```python
from build123d import *

# Parameters (mm, degrees)
BOSS_EXTRUDE1_DEPTH         = 35
CUT_EXTRUDE1_REACH          = 51.749
SKETCH2_R                   = 18
CUT_EXTRUDE2_DEPTH          = 22
CUT_EXTRUDE3_DEPTH          = 16
SKETCH5_W                   = 4.5
SKETCH5_H                   = 3
CUT_REVOLVE1_ANGLE          = 120
FILLET2_R                   = 1.5
CUT_EXTRUDE7_DEPTH          = 6.5
M3X0_25_TAPPED_HOLE1_REACH  = 71.769
M3X0_25_TAPPED_HOLE1_BORE_R = 1.375
M3X0_25_TAPPED_HOLE2_REACH  = 71.769
M3X0_25_TAPPED_HOLE2_BORE_R = 1.375
CUT_EXTRUDE8_REACH          = 71.769
CUT_EXTRUDE8_END_RADIUS     = 18
SKETCH15_R                  = 1.6
CUT_EXTRUDE9_REACH          = 71.769
CUT_EXTRUDE9_END_RADIUS     = 18
SKETCH16_R                  = 1.6
M5_TAPPED_HOLE3_D           = 4.2
M5_TAPPED_HOLE3_DEPTH       = 4.3
M5_TAPPED_HOLE3_TIP         = 1.2618073
M5_TAPPED_HOLE4_D           = 4.2
M5_TAPPED_HOLE4_DEPTH       = 4.3
M5_TAPPED_HOLE4_TIP         = 1.2618073
M3_TAPPED_HOLE1_D           = 2.5
M3_TAPPED_HOLE1_DEPTH       = 11.5
M3_TAPPED_HOLE1_TIP         = 0.751075774
FILLET3_R                   = 1.5


with BuildPart() as part:
    # Sketch1 → Boss-Extrude1 (new body)
    with BuildSketch(Plane(origin=(0, 0, 0), x_dir=(1, 0, 0), z_dir=(0, 1, 0))):
        Polygon((10.355339059, 25), (-10.355339059, 25), (-25, 10.355339059), (-25, -10.355339059), (-10.355339059, -25), (10.355339059, -25), (25, -10.355339059), (25, 10.355339059), align=None)
    extrude(amount=BOSS_EXTRUDE1_DEPTH)

    # Sketch2 → Cut-Extrude1 (cut, up to next)
    with BuildSketch(Plane(origin=(0, 35, 0), x_dir=(1, 0, 0), z_dir=(0, 1, 0)), mode=Mode.PRIVATE) as cut_extrude1_sk1:
        with Locations(Location((0, 0, 0), (0, 0, 270))):
            Circle(SKETCH2_R)
    cut_extrude1_tool1 = extrude(cut_extrude1_sk1.sketch, amount=-CUT_EXTRUDE1_REACH, mode=Mode.PRIVATE) & part.part
    add(cut_extrude1_tool1.solids().sort_by_distance((0, 35, 0))[0], mode=Mode.SUBTRACT)

    # Sketch3 → Cut-Extrude2 (cut)
    with BuildSketch(Plane(origin=(0, 35, 0), x_dir=(1, 0, 0), z_dir=(0, 1, 0))):
        with BuildLine():
            Line((-10.355339059, 25), (-17.677669284, 17.677669776))
            ThreePointArc((-17.677669284, 17.677669776), (-9.567085631, 23.096988387), (3.8e-08, 25))
            Line((3.8e-08, 25), (-10.355339059, 25))
        make_face()
        with BuildLine():
            Line((-17.677669284, 17.677669776), (-25, 10.355339059))
            Line((-25, 10.355339059), (-22.754493028, 10.355339059))
            ThreePointArc((-22.754493028, 10.355339059), (-20.544928062, 14.244505289), (-17.677669284, 17.677669776))
        make_face()
        with BuildLine():
            Line((10.355339059, 25), (3.8e-08, 25))
            ThreePointArc((3.8e-08, 25), (9.56708591, 23.096988271), (17.677669657, 17.677669402))
            Line((17.677669657, 17.677669402), (10.355339059, 25))
        make_face()
        with BuildLine():
            Line((25, 10.355339059), (17.677669657, 17.677669402))
            ThreePointArc((17.677669657, 17.677669402), (20.544928213, 14.244505072), (22.754493028, 10.355339059))
            Line((22.754493028, 10.355339059), (25, 10.355339059))
        make_face()
    extrude(amount=-CUT_EXTRUDE2_DEPTH, mode=Mode.SUBTRACT)

    # Sketch4 → Cut-Extrude3 (cut)
    with BuildSketch(Plane(origin=(0, 35, 0), x_dir=(1, 0, 0), z_dir=(0, 1, 0))):
        with BuildLine():
            Line((-16.38323498, 7.455844123), (-22.754493028, 10.355339059))
            ThreePointArc((-22.754493028, 10.355339059), (0, 25), (22.754493028, 10.355339059))
            Line((22.754493028, 10.355339059), (16.38323498, 7.455844123))
            ThreePointArc((16.38323498, 7.455844123), (0, 18), (-16.38323498, 7.455844123))
        make_face()
    extrude(amount=-CUT_EXTRUDE3_DEPTH, mode=Mode.SUBTRACT)

    # Sketch5 → Cut-Revolve1 (revolve, symmetric, cut)
    with BuildSketch(Plane(origin=(0, 0, 0), x_dir=(0, 0, -1), z_dir=(1, 0, 0))) as cut_revolve1_sk:
        with Locations((22.75, 15.5)):
            Rectangle(SKETCH5_W, SKETCH5_H)
    revolve(axis=Axis((0, 0, 0), (0, 1, 0)), revolution_arc=CUT_REVOLVE1_ANGLE / 2, mode=Mode.SUBTRACT)
    revolve(cut_revolve1_sk.sketch, axis=Axis((0, 0, 0), (0, -1, 0)), revolution_arc=CUT_REVOLVE1_ANGLE / 2, mode=Mode.SUBTRACT)

    # Fillet2
    fillet2_edges = [part.edges().sort_by_distance(p)[0] for p in [
        (19.702077936, 14, -11.375),
        (19.702077936, 17, -11.375),
        (-19.702077936, 17, -11.375),
        (-19.702077936, 14, -11.375),
    ]]
    fillet(fillet2_edges, radius=FILLET2_R - 0.0001)  # a hair under: the kernel refuses the full size

    # Sketch9 → Cut-Extrude7 (cut)
    with BuildSketch(Plane(origin=(0, 19, 0), x_dir=(1, 0, 0), z_dir=(0, 1, 0))):
        with BuildLine():
            ThreePointArc((20.178391908, 11.65), (0, 23.3), (-20.178391908, 11.65))
            ThreePointArc((-20.178391908, 11.65), (-19.574449992, 9.396058084), (-17.320508076, 10))
            ThreePointArc((-17.320508076, 10), (0, 20), (17.320508076, 10))
            ThreePointArc((17.320508076, 10), (19.574449992, 9.396058084), (20.178391908, 11.65))
        make_face()
    extrude(amount=-CUT_EXTRUDE7_DEPTH, mode=Mode.SUBTRACT)

    # M3x0.25 Tapped Hole1 bore → M3x0.25 Tapped Hole1 (cut, up to next)
    with BuildSketch(Plane(origin=(-17.67766953, 0, -17.67766953), x_dir=(-0.7071067811865472, 0, 0.7071067811865479), z_dir=(-0.7071067811865479, 0, -0.7071067811865472)), mode=Mode.PRIVATE) as m3x0_25_tapped_hole1_sk1:
        with Locations((0, 7.5)):
            Circle(M3X0_25_TAPPED_HOLE1_BORE_R)
    m3x0_25_tapped_hole1_tool1 = extrude(m3x0_25_tapped_hole1_sk1.sketch, amount=-M3X0_25_TAPPED_HOLE1_REACH, mode=Mode.PRIVATE) & part.part
    add(m3x0_25_tapped_hole1_tool1.solids().sort_by_distance((-17.67767, 7.5, -17.67767))[0], mode=Mode.SUBTRACT)

    # M3x0.25 Tapped Hole2 bore → M3x0.25 Tapped Hole2 (cut, up to next)
    with BuildSketch(Plane(origin=(17.67766953, 0, -17.67766953), x_dir=(-0.7071067811865475, 0, -0.7071067811865477), z_dir=(0.7071067811865477, 0, -0.7071067811865475)), mode=Mode.PRIVATE) as m3x0_25_tapped_hole2_sk1:
        with Locations((0, 7.5)):
            Circle(M3X0_25_TAPPED_HOLE2_BORE_R)
    m3x0_25_tapped_hole2_tool1 = extrude(m3x0_25_tapped_hole2_sk1.sketch, amount=-M3X0_25_TAPPED_HOLE2_REACH, mode=Mode.PRIVATE) & part.part
    add(m3x0_25_tapped_hole2_tool1.solids().sort_by_distance((17.67767, 7.5, -17.67767))[0], mode=Mode.SUBTRACT)

    # Cut-Extrude8: up to this cylinder (the profile starts outside it)
    cut_extrude8_end = Plane(origin=(0, 7.5, 0), z_dir=(0, 1, 0)) * Cylinder(CUT_EXTRUDE8_END_RADIUS, 180.538, mode=Mode.PRIVATE)
    # Sketch15 → Cut-Extrude8 (cut, up to the surface)
    with BuildSketch(Plane(origin=(17.67766953, 0, 17.67766953), x_dir=(0.7071067811865472, 0, -0.7071067811865479), z_dir=(0.7071067811865479, 0, 0.7071067811865472)), mode=Mode.PRIVATE) as cut_extrude8_sk1:
        with Locations((0, 7.5)):
            Circle(SKETCH15_R)
    cut_extrude8_tool1 = extrude(cut_extrude8_sk1.sketch, amount=-CUT_EXTRUDE8_REACH, mode=Mode.PRIVATE) - cut_extrude8_end
    add(cut_extrude8_tool1.solids().sort_by_distance((17.67767, 7.5, 17.67767))[0], mode=Mode.SUBTRACT)

    # Cut-Extrude9: up to this cylinder (the profile starts outside it)
    cut_extrude9_end = Plane(origin=(0, 7.5, 0), z_dir=(0, 1, 0)) * Cylinder(CUT_EXTRUDE9_END_RADIUS, 180.538, mode=Mode.PRIVATE)
    # Sketch16 → Cut-Extrude9 (cut, up to the surface)
    with BuildSketch(Plane(origin=(-17.67766953, 0, 17.67766953), x_dir=(0.7071067811865477, 0, 0.7071067811865475), z_dir=(-0.7071067811865475, 0, 0.7071067811865477)), mode=Mode.PRIVATE) as cut_extrude9_sk1:
        with Locations((0, 7.5)):
            Circle(SKETCH16_R)
    cut_extrude9_tool1 = extrude(cut_extrude9_sk1.sketch, amount=-CUT_EXTRUDE9_REACH, mode=Mode.PRIVATE) - cut_extrude9_end
    add(cut_extrude9_tool1.solids().sort_by_distance((-17.67767, 7.5, 17.67767))[0], mode=Mode.SUBTRACT)

    # M5 Tapped Hole3
    with Locations(Plane(origin=(-17.67766953, 0, 17.67766953), x_dir=(0.7071067811865477, 0, 0.7071067811865475), z_dir=(-0.7071067811865475, 0, 0.7071067811865477))):
        with Locations((0, 7.5)):
            Hole(M5_TAPPED_HOLE3_D / 2, depth=M5_TAPPED_HOLE3_DEPTH)
            with Locations((0, 0, -(M5_TAPPED_HOLE3_DEPTH + M5_TAPPED_HOLE3_TIP / 2))):  # 118° drill point
                Cone(0, M5_TAPPED_HOLE3_D / 2, M5_TAPPED_HOLE3_TIP, mode=Mode.SUBTRACT)

    # M5 Tapped Hole4
    with Locations(Plane(origin=(17.67766953, 0, 17.67766953), x_dir=(0.7071067811865472, 0, -0.7071067811865479), z_dir=(0.7071067811865479, 0, 0.7071067811865472))):
        with Locations((0, 7.5)):
            Hole(M5_TAPPED_HOLE4_D / 2, depth=M5_TAPPED_HOLE4_DEPTH)
            with Locations((0, 0, -(M5_TAPPED_HOLE4_DEPTH + M5_TAPPED_HOLE4_TIP / 2))):  # 118° drill point
                Cone(0, M5_TAPPED_HOLE4_D / 2, M5_TAPPED_HOLE4_TIP, mode=Mode.SUBTRACT)

    # M3 Tapped Hole1
    with Locations(Plane(origin=(0, 35, 0), x_dir=(1, 0, 0), z_dir=(0, 1, 0))):
        with Locations((-21.25, 7.395099729), (21.25, 7.395099729), (-8, -21.029740845), (8, -21.029740845)):
            Hole(M3_TAPPED_HOLE1_D / 2, depth=M3_TAPPED_HOLE1_DEPTH)
            with Locations((0, 0, -(M3_TAPPED_HOLE1_DEPTH + M3_TAPPED_HOLE1_TIP / 2))):  # 118° drill point
                Cone(0, M3_TAPPED_HOLE1_D / 2, M3_TAPPED_HOLE1_TIP, mode=Mode.SUBTRACT)

    # Fillet3
    fillet3_edges = [part.edges().sort_by_distance(p)[0] for p in [
        (22.754493028, 16, -10.355339059),
        (-22.754493028, 16, -10.355339059),
    ]]
    fillet(fillet3_edges, radius=FILLET3_R)


solid = part.part
```
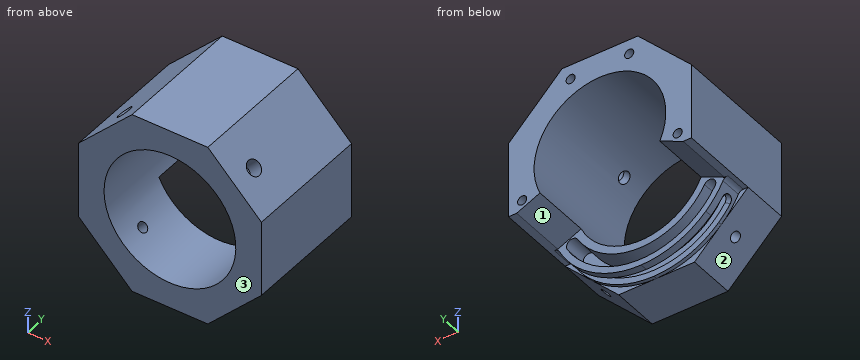
Could you check a few things on this model? Use its own coordinates, in mm. Face numbers are marked on the shaded views. Round coordinates to 2 decimals unless told otherwise and drop trailing zeros. Loops run counter-clockwise (first coordinate to the right, second up) from the corner with the lowest first, then second, coordinate; pieces in that order, holes last.
Q1. I want a section at A-A (y = 10.5). Write out the boundary of the cut face in (x, z).
Q2. I want a section at C-C (x = 3.5). Write out the boundary of the cut face in (y, z).
Q3. Please list where these lines run through material, in increasing order: L1, parallel to Z at x = -1.5, y = 17.5; L2, parallel to Z at x = 8, y = 31; L3, parallel to X at y = 24.5, z = -8.
Q4. For P1, Ø8, axis at x = -22, z = -15, coming from the +Y side; P2, Ø1.5, axis at x = -11.5, y = 19, coming from the -Z side; P3, Ø1.1, axis at x = 24.5, y = 22.5, coming from the -Z side, each with a flat end and sliding along its axis, tell me the tip position at first contact or that it passes through.
Q5. I want a section at B-B (z = 0). Write out the boundary of the cut face in (x, y), and give its area (3 significant figures).
Q6. I want a section at D-D (y = 27). Write out the boundary of the cut face in (x, z), and give its area (3 significant figures).
Q7. Thinking about a two-plate mould opening in X: for the marked faces 1, 2 and 3, which applies, pulls with the +X half, pulls with the -X half, needs draft (parallel to the pull), parting line crosses it, or undercut?
Answer below:
1. outline: (-25, -10.36) - (-10.36, -25) - (10.36, -25) - (25, -10.36) - (25, 10.36) - (10.36, 25) - (-10.36, 25) - (-25, 10.36) - close; hole circle Ø36 at (0, 0)
2. outline: (0, -25) - (13, -25) - (13, -24.75) - (14, -24.75) - (14, -23.04) - (12.5, -23.04) - (12.5, -19.69) - (19, -19.69) - (19, -17.66) - (0, -17.66) - close; (0, 17.66) - (35, 17.66) - (35, 25) - (0, 25) - close; (17, -24.75) - (19, -24.75) - (19, -23.04) - (17, -23.04) - close
3. L1: z = -24.95 to -23.25, -19.94 to -17.94, 17.94 to 25
3. L2: z = 16.12 to 19.78, 22.28 to 25
3. L3: x = -25 to -22.34, -20.16 to -17.58, 17.58 to 20.16, 22.34 to 25
4. P1: stops at y = 19
4. P2: stops at z = -22.57
4. P3: stops at z = -10.36
5. outline: (-25, 0) - (-18, 0) - (-18, 35) - (-25, 35) - close; (18, 0) - (25, 0) - (25, 35) - (18, 35) - close
5. area: 490 mm2
6. outline: (-25, -10.36) - (-22.75, -10.36) - (-16.38, -7.46) arc R18 cw (long way) to (16.38, -7.46) - (22.75, -10.36) - (25, -10.36) - (25, 10.36) - (10.36, 25) - (-10.36, 25) - (-25, 10.36) - close; hole circle Ø2.5 at (-21.25, -7.4); hole circle Ø2.5 at (-8, 21.03); hole circle Ø2.5 at (8, 21.03); hole circle Ø2.5 at (21.25, -7.4)
6. area: 651 mm2
7. face 1: undercut
7. face 2: pulls with the -X half
7. face 3: needs draft
